from build123d import *
from OCP.BRepFilletAPI import BRepFilletAPI_MakeChamfer

# Parameters (mm, degrees)
SKETCH1_W           = 14
SKETCH1_H           = 14.2
BOSS_EXTRUDE2_DEPTH = 5.5
SKETCH2_W           = 1
SKETCH2_H           = 2.5
CUT_EXTRUDE1_DEPTH  = 2.5
SKETCH3_W           = 1.5
SKETCH3_H           = 2.5
CUT_EXTRUDE2_DEPTH  = 3
SKETCH4_W           = 0.5
SKETCH4_H           = 6.5
CUT_EXTRUDE3_DEPTH  = 5.5
SKETCH5_W           = 1
SKETCH5_H           = 4.5
CUT_EXTRUDE4_DEPTH  = 4.5
CHAMFER2_SIZE       = 1.75
CHAMFER2_SIZE2      = 0.63694791
CHAMFER3_SIZE       = 1.75
CHAMFER3_SIZE2      = 0.63694791
SKETCH7_W           = 9.72610418
SKETCH7_H           = 2.85
CUT_EXTRUDE5_DEPTH  = 21.685502169
SKETCH8_W           = 9.72610418
SKETCH8_H           = 8.35
CUT_EXTRUDE6_DEPTH  = 5
CHAMFER4_SIZE       = 0.5
CHAMFER4_SIZE2      = 2.83564091
CHAMFER5_SIZE       = 0.5
CHAMFER5_SIZE2      = 2.83564091
SKETCH9_W           = 14
SKETCH9_H           = 0.5
CUT_EXTRUDE7_DEPTH  = 5
SKETCH11_W          = 2
SKETCH11_H          = 0.5
CUT_EXTRUDE11_DEPTH = 2
FILLET2_R           = 0.5
CUT_EXTRUDE12_START = -3.35
SKETCH12_W          = 9.73
SKETCH12_H          = 2
CUT_EXTRUDE12_DEPTH = 3.35
SKETCH13_W          = 0.5
SKETCH13_H          = 0.713041147
SKETCH13_W_2        = 0.385
SKETCH13_H_2        = 5
BOSS_EXTRUDE3_DEPTH = 0.2
FILLET4_R           = 0.5


with BuildPart() as part:
    # Sketch1 → Boss-Extrude2 (new body)
    with BuildSketch(Plane(origin=(0, 0, 0), x_dir=(1, 0, 0), z_dir=(0, 1, 0))):
        with Locations((-7, 7.1)):
            Rectangle(SKETCH1_W, SKETCH1_H)
    extrude(amount=-BOSS_EXTRUDE2_DEPTH)

    # Sketch2 → Cut-Extrude1 (cut)
    with BuildSketch(Plane(origin=(0, 0, 0), x_dir=(1, 0, 0), z_dir=(0, 1, 0))):
        with Locations((-13.5, 11.6)):
            Rectangle(SKETCH2_W, SKETCH2_H)
        with Locations((-0.5, 11.6)):
            Rectangle(SKETCH2_W, SKETCH2_H)
        with Locations((-13.5, 2.6)):
            Rectangle(SKETCH2_W, SKETCH2_H)
        with Locations((-0.5, 2.6)):
            Rectangle(SKETCH2_W, SKETCH2_H)
    extrude(amount=-CUT_EXTRUDE1_DEPTH, mode=Mode.SUBTRACT)

    # Sketch3 → Cut-Extrude2 (cut)
    with BuildSketch(Plane.XZ.offset(5.5)):
        with Locations((-13.25, -2.6)):
            Rectangle(SKETCH3_W, SKETCH3_H)
        with Locations((-0.75, -2.6)):
            Rectangle(SKETCH3_W, SKETCH3_H)
        with Locations((-0.75, -11.6)):
            Rectangle(SKETCH3_W, SKETCH3_H)
        with Locations((-13.25, -11.6)):
            Rectangle(SKETCH3_W, SKETCH3_H)
    extrude(amount=-CUT_EXTRUDE2_DEPTH, mode=Mode.SUBTRACT)

    # Sketch4 → Cut-Extrude3 (cut)
    with BuildSketch(Plane(origin=(0, 0, 0), x_dir=(1, 0, 0), z_dir=(0, 1, 0))):
        with Locations((-0.25, 7.1)):
            Rectangle(SKETCH4_W, SKETCH4_H)
        with Locations((-13.75, 7.1)):
            Rectangle(SKETCH4_W, SKETCH4_H)
    extrude(amount=-CUT_EXTRUDE3_DEPTH, mode=Mode.SUBTRACT)

    # Sketch5 → Cut-Extrude4 (cut)
    with BuildSketch(Plane(origin=(0, 0, 0), x_dir=(1, 0, 0), z_dir=(0, 1, 0))):
        with Locations((-13, 7.1)):
            Rectangle(SKETCH5_W, SKETCH5_H)
        with Locations((-1, 7.1)):
            Rectangle(SKETCH5_W, SKETCH5_H)
    extrude(amount=-CUT_EXTRUDE4_DEPTH, mode=Mode.SUBTRACT)

    # Chamfer2: one chamfer whose edges measure the first distance from different faces: ONE call of the kernel's chamfer builder (chamfer() names one face for all edges)
    chamfer2_edges_1 = [part.edges().sort_by_distance(p)[0] for p in [
        (-13, 0, -2.6),
    ]]
    chamfer2_side_1 = [part.faces().sort_by_distance(p)[0] for p in [
        (-13, -1.25, -2.6),
    ]]
    chamfer2_edges_2 = [part.edges().sort_by_distance(p)[0] for p in [
        (-13, 0, -11.6),
    ]]
    chamfer2_side_2 = [part.faces().sort_by_distance(p)[0] for p in [
        (-13, -1.25, -11.6),
    ]]
    chamfer2 = BRepFilletAPI_MakeChamfer(part.part.solid().wrapped)
    for e in chamfer2_edges_1:
        chamfer2.Add(CHAMFER2_SIZE, CHAMFER2_SIZE2, e.wrapped, chamfer2_side_1[0].wrapped)  # the first distance lies on this face
    for e in chamfer2_edges_2:
        chamfer2.Add(CHAMFER2_SIZE, CHAMFER2_SIZE2, e.wrapped, chamfer2_side_2[0].wrapped)  # the first distance lies on this face
    add(Compound.cast(chamfer2.Shape()), mode=Mode.REPLACE)

    # Chamfer3: one chamfer whose edges measure the first distance from different faces: ONE call of the kernel's chamfer builder (chamfer() names one face for all edges)
    chamfer3_edges_1 = [part.edges().sort_by_distance(p)[0] for p in [
        (-1, 0, -11.6),
    ]]
    chamfer3_side_1 = [part.faces().sort_by_distance(p)[0] for p in [
        (-1, -1.25, -11.6),
    ]]
    chamfer3_edges_2 = [part.edges().sort_by_distance(p)[0] for p in [
        (-1, 0, -2.6),
    ]]
    chamfer3_side_2 = [part.faces().sort_by_distance(p)[0] for p in [
        (-1, -1.25, -2.6),
    ]]
    chamfer3 = BRepFilletAPI_MakeChamfer(part.part.solid().wrapped)
    for e in chamfer3_edges_1:
        chamfer3.Add(CHAMFER3_SIZE, CHAMFER3_SIZE2, e.wrapped, chamfer3_side_1[0].wrapped)  # the first distance lies on this face
    for e in chamfer3_edges_2:
        chamfer3.Add(CHAMFER3_SIZE, CHAMFER3_SIZE2, e.wrapped, chamfer3_side_2[0].wrapped)  # the first distance lies on this face
    add(Compound.cast(chamfer3.Shape()), mode=Mode.REPLACE)

    # Sketch7 → Cut-Extrude5 (cut, through all)
    with BuildSketch(Plane(origin=(0, 0, 0), x_dir=(1, 0, 0), z_dir=(0, 1, 0))):
        with Locations((-7, 2.425)):
            Rectangle(SKETCH7_W, SKETCH7_H)
    extrude(amount=-CUT_EXTRUDE5_DEPTH, mode=Mode.SUBTRACT)

    # Sketch8 → Cut-Extrude6 (cut)
    with BuildSketch(Plane(origin=(0, 0, 0), x_dir=(1, 0, 0), z_dir=(0, 1, 0))):
        with Locations((-7, 8.525)):
            Rectangle(SKETCH8_W, SKETCH8_H)
    extrude(amount=-CUT_EXTRUDE6_DEPTH, mode=Mode.SUBTRACT)

    # Chamfer4
    chamfer4_edges = [part.edges().sort_by_distance(p)[0] for p in [
        (0, -5.5, -0.675),
        (0, -5.5, -13.525),
    ]]
    chamfer4_side = [part.faces().sort_by_distance(p)[0] for p in [
        (-7, -5.5, -7.966343482),
    ]]
    chamfer(chamfer4_edges, length=CHAMFER4_SIZE, length2=CHAMFER4_SIZE2, reference=chamfer4_side[0])

    # Chamfer5
    chamfer5_edges = [part.edges().sort_by_distance(p)[0] for p in [
        (-14, -5.5, -13.525),
        (-14, -5.5, -0.675),
    ]]
    chamfer5_side = [part.faces().sort_by_distance(p)[0] for p in [
        (-7.06147516, -5.5, -7.974233646),
    ]]
    chamfer(chamfer5_edges, length=CHAMFER5_SIZE, length2=CHAMFER5_SIZE2, reference=chamfer5_side[0])

    # Sketch9 → Cut-Extrude7 (cut)
    with BuildSketch(Plane.XZ.offset(5.5)):
        with Locations((-7, -0.25)):
            Rectangle(SKETCH9_W, SKETCH9_H)
        with Locations((-7, -13.95)):
            Rectangle(SKETCH9_W, SKETCH9_H)
    extrude(amount=-CUT_EXTRUDE7_DEPTH, mode=Mode.SUBTRACT)

    # Sketch11 → Cut-Extrude11 (cut)
    with BuildSketch(Plane(origin=(0, 0, 0), x_dir=(1, 0, 0), z_dir=(0, 1, 0))):
        with Locations((-9.5, 0.75)):
            Rectangle(SKETCH11_W, SKETCH11_H)
        Polygon((-10.5, 0.5), (-10.5, 0), (-3.5, 0), (-3.5, 0.5), (-5.5, 0.5), (-8.5, 0.5), align=None)
        with Locations((-4.5, 0.75)):
            Rectangle(SKETCH11_W, SKETCH11_H)
    extrude(amount=-CUT_EXTRUDE11_DEPTH, mode=Mode.SUBTRACT)

    # Fillet2
    fillet2_edges = [part.edges().sort_by_distance(p)[0] for p in [
        (-10.5, -2, -0.75),
        (-5.5, -2, -0.75),
        (-3.5, -2, -0.75),
        (-8.5, -2, -0.75),
    ]]
    fillet(fillet2_edges, radius=FILLET2_R)

    # Sketch12 → Cut-Extrude12 (cut)
    with BuildSketch(Plane.XY.offset(-0.5).offset(CUT_EXTRUDE12_START)):
        with Locations((-7, -4.5)):
            Rectangle(SKETCH12_W, SKETCH12_H)
    extrude(amount=CUT_EXTRUDE12_DEPTH, mode=Mode.SUBTRACT)

    # Sketch13 → Boss-Extrude3 (add)
    with BuildSketch(Plane.XY.offset(-0.5)):
        with Locations((-7.5, -2.158926418)):
            Rectangle(SKETCH13_W, SKETCH13_H)
        with Locations((-6.5, -2.158926418)):
            Rectangle(SKETCH13_W, SKETCH13_H)
        with Locations((-1.9425, -3)):
            Rectangle(SKETCH13_W_2, SKETCH13_H_2)
        with Locations((-12.0575, -3)):
            Rectangle(SKETCH13_W_2, SKETCH13_H_2)
    extrude(amount=BOSS_EXTRUDE3_DEPTH)

    # Fillet4
    # the kernel refuses this fillet: 0.5 mm, written as the material it takes off along each edge
    with BuildSketch(Plane(origin=(-8.75, -1.802405844, -0.3), x_dir=(0, -2.6074697955836492e-11, -1.0), z_dir=(1, 0, 0)), Plane(origin=(-7.75, -1.802405844, -0.3), x_dir=(0, -2.6074697955836492e-11, -1.0), z_dir=(1, 0, 0))) as fillet4_piece_1:
        with BuildLine():
            CenterArc((0.5, -0.4), FILLET4_R, 126.869897647, 53.130102355)
            Line((0, -0.4), (-0.01, -0.4))
            Line((-0.01, -0.4), (-0.01, 0))
            Line((-0.01, 0), (0, 0.01))
            ThreePointArc((0, 0.01), (0.1, 0.01), (0.194, 0.008))
            Line((0.194, 0.008), (0.2, 0))
        make_face()
    extrude(amount=2.5, mode=Mode.SUBTRACT)
    with BuildSketch(Plane(origin=(-5.25, -2.515446991, -0.3), x_dir=(0, 1, 0), z_dir=(-1, 0, 0)), Plane(origin=(-6.25, -2.515446991, -0.3), x_dir=(0, 1, 0), z_dir=(-1, 0, 0))) as fillet4_piece_2:
        with BuildLine():
            CenterArc((0.4, 0.5), FILLET4_R, 216.869897645, 53.130102355)
            Line((0, 0.2), (-0.008, 0.194))
            ThreePointArc((-0.008, 0.194), (-0.01, 0.1), (-0.01, 0))
            Line((-0.01, 0), (0, -0.01))
            Line((0, -0.01), (0.4, -0.01))
            Line((0.4, -0.01), (0.4, 0))
        make_face()
    extrude(amount=2.5, mode=Mode.SUBTRACT)


solid = part.part
Verification items for the finished model (mm, model axes). A direction names the side the tool comes from. Give positions to 0.01 mm unless a question says otherwise; leave off trailing zeros. Loops run counter-clockwise (first coordinate to the right, second up) from the corner with the lowest first, then second, coordinate; pieces in that order, holes last.
1) Sectioned sample at D-D, the plane z = -6.25. Enter the section's corners in (x, y), then the cut area to 3 significant figures.
2) Set-up check for faces 1 (the flat face through (-2.137, -2, -2)), 2 (the flat face through (-1, -4.5, -7)), 3 (the flat face through (-2.137, -2, -8)), 4 (the flat face through (-13, -3, -10.35)), 5 (the flat face through (-12.677, -0.863, -2.583)): record each of +Z, -Z, +X, -X, +Y, -Y from which the full face is reachable in a straight line by a thin tool's end or side.
3) Thickness scan on line 1 along Z through (x, y) = (-3, -1.45); line 2 along Z through (x, y) = (-1, -1.4); line 3 along X through (y, z) = (-2.6, -12). Record the ranges inside material, lowest first.
4) Sectioned sample at A-A, the plane x = -3.25. Enter the section's corners in (y, z), then the cut area to 3 significant figures.
5) Draft check along Z on faces 6 (the flat face through (-7, -3, -13.7)), 7 (the flat face through (-7, -2, -1)), 8 (the flat face through (0, -1, -13)). Enter one of: pulls with the +Z half, pulls with the -Z half, needs draft (parallel to the pull), parting line crosses it, or undercut.
6) Depth check by flat-ended pin: pin 1 Ø1.5 at (x, z) = (-4, -6) entering from +Y; pin 2 Ø1.8 at (x, y) = (-1, -4) entering from +Z; pin 3 Ø1 at (x, z) = (-3.5, -2.5) entering from -Y; pin 4 Ø0.5 at (x, y) = (-1, -2.5) entering from -Z. Enter the tip coordinate at first touch or a pass-through.
7) Sectioned sample at C-C, the plane x = -8. Enter the section's corners in (y, z), then the cut area to 3 significant figures.
Answers:
1. outline: (-13.5, -5.5) - (-0.5, -5.5) - (-0.5, -4.5) - (-1.5, -4.5) - (-1.5, 0) - (-2.14, 0) - (-2.14, -5) - (-11.86, -5) - (-11.86, 0) - (-12.5, 0) - (-12.5, -4.5) - (-13.5, -4.5) - close
1. area: 13.9 mm2
2. face 1: +Y, -Y
2. face 2: +X, +Y
2. face 3: +Y
2. face 4: -X
2. face 5: -X, +Y
3. line 1: z = -13.7 to -12.7, -4.35 to -3.85, -1 to -0.5
3. line 2: z = -13.7 to -12.85, -10.35 to -9.35, -4.85 to -3.85, -1.35 to -0.5
3. line 3: x = -12.5 to -11.86, -2.14 to -1.5
4. outline: (-5.5, -13.7) - (-0.5, -13.7) - (-0.5, -14.2) - (0, -14.2) - (0, -12.7) - (-5, -12.7) - (-5, -4.35) - (0, -4.35) - (0, -3.85) - (-5.5, -3.85) - close; (-3.5, -1) - (0, -1) - (0, 0) - (-0.5, 0) - (-0.5, -0.5) - (-3.5, -0.5) - close
4. area: 14.7 mm2
5. face 6: pulls with the -Z half
5. face 7: undercut
5. face 8: needs draft
6. pin 1: stops at y = -5
6. pin 2: stops at z = -0.3
6. pin 3: passes through
6. pin 4: stops at z = -13.7
7. outline: (-5.5, -13.7) - (-0.5, -13.7) - (-0.5, -14.2) - (0, -14.2) - (0, -12.7) - (-5, -12.7) - (-5, -4.35) - (0, -4.35) - (0, -3.85) - (-5.5, -3.85) - close; (-3.5, -1) - (0, -1) - (0, -0.5) - (-3.5, -0.5) - close
7. area: 14.4 mm2
